Read the model definition and answer for the solid it produces. Units are mm, in the model's axes. Face numbers are marked on the shaded views. A direction names the side the tool comes from. Coordinates: 2 decimals unless noted, no trailing zeros. Loops run counter-clockwise (first coordinate to the right, second up) from the corner with the lowest first, then second, coordinate; pieces in that order, holes last. Notation, with made-up numbers: (62.5, 59) - (93.5, 59) arc R31 cw to (93.5, 91) - close; hole circle Ø8 at (35.5, -14.75). An arc over 180 degrees is marked (long way). Use one line per item in the form item = value. Start each with the question number.
1) A cutting plane is placed at D-D (x = 4). Give the vertices of the cut face in (y, z).
2) Each of these flat-tipped pins is pushed along its axis until it touches: P1, Ø2, axis at x = 0, z = 6, coming from the -Y side; P2, Ø1, axis at x = 9, y = 0, coming from the -Z side. Where does it stop, or does it pass through?
3) A cutting plane is placed at A-A (y = 3). Give the vertices of the cut face in (x, z).
4) A cutting plane is placed at B-B (x = 9). Give the vertices of the cut face in (y, z), and give its area (3 significant figures).
5) A cutting plane is placed at C-C (x = -1.25). Give the vertices of the cut face in (y, z).
6) Which of the six approach directions +Z, -Z, +X, -X, +Y, -Y give full straight-line access (tool end or side, diameter ignored) to the marked faces 1, 2, 3, 4 and 5?
7) The mould has two halves that part along X. Classify the marked faces 6, 7, 8 and 9: released by +X, released by -X, zero draft, split by the parting line, or undercut.
8) Consider line 1 (Y direction, x = 5.25, z = 6.75); line 2 (X direction, y = 3, z = 6.75); line 3 (Z direction, x = 1.75, y = -1). Determine where each line is inside the solid, lowest interval first.
from build123d import *

# Parameters (mm, degrees)
SKETCH1_W           = 12
SKETCH1_H           = 6
BOSS_EXTRUDE1_DEPTH = 7
SKETCH2_R           = 3
BOSS_EXTRUDE2_DEPTH = 2.5
SKETCH3_R           = 0.5
BOSS_EXTRUDE3_DEPTH = 2.1
FILLET1_R           = 0.5


with BuildPart() as part:
    # Sketch1 → Boss-Extrude1 (new body)
    with BuildSketch(Plane.XY):
        with Locations((6, 3)):
            Rectangle(SKETCH1_W, SKETCH1_H)
    extrude(amount=BOSS_EXTRUDE1_DEPTH)

    # Sketch2 → Boss-Extrude2 (add)
    with BuildSketch(Plane.ZY):
        with Locations(Location((3.5, 3, 0), (0, 0, 270))):
            Circle(SKETCH2_R)
    extrude(amount=BOSS_EXTRUDE2_DEPTH)

    # Sketch3 → Boss-Extrude3 (add)
    with BuildSketch(Plane.XZ):
        with Locations(Location((2, 3.5, 0), (0, 0, 90))):
            Circle(SKETCH3_R)
        with Locations(Location((9, 3.5, 0), (0, 0, 90))):
            Circle(SKETCH3_R)
    extrude(amount=BOSS_EXTRUDE3_DEPTH)

    # Fillet1
    fillet1_edges = [part.edges().sort_by_distance(p)[0] for p in [
        (2, -2.1, 3),
        (9, -2.1, 3),
    ]]
    fillet(fillet1_edges, radius=FILLET1_R)


solid = part.part
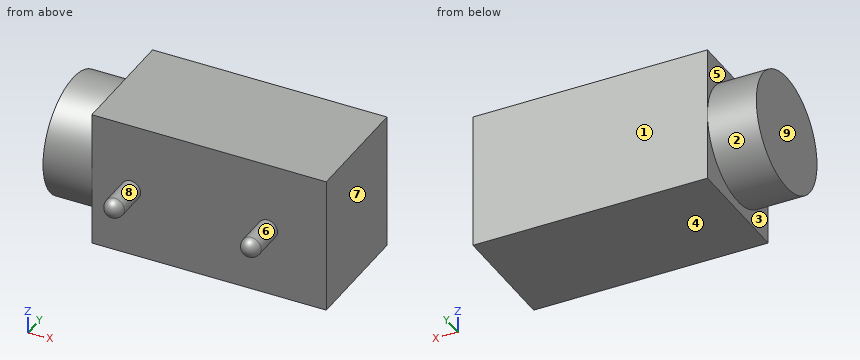
Found:
q1.outline = (0, 0) - (6, 0) - (6, 7) - (0, 7) - close
q2.P1 = 0
q2.P2 = 0
q3.outline = (-2.5, 0.5) - (0, 0.5) - (0, 0) - (12, 0) - (12, 7) - (0, 7) - (0, 6.5) - (-2.5, 6.5) - close
q4.outline = (-1.6, 3) - (0, 3) - (0, 0) - (6, 0) - (6, 7) - (0, 7) - (0, 4) - (-1.6, 4) arc R0.5 ccw to start
q4.area = 44.0 mm^2
q5.outline = circle Ø6 at (3, 3.5)
q6.face_1 = +Z, -Z, +X, -X, +Y
q6.face_2 = -X
q6.face_3 = -Z, -X
q6.face_4 = -Z, +X, -X, +Y, -Y
q6.face_5 = +Z, -X
q7.face_6 = undercut
q7.face_7 = released by +X
q7.face_8 = undercut
q7.face_9 = released by -X
q8.line_1 = 0 to 6
q8.line_2 = 0 to 12
q8.line_3 = 3.07 to 3.93
